Check sheet for the drawn part. Datum: minimum x, y, z corner. Units: mm. A direction names the side the tool comes from. Coordinates: 2 decimals unless noted, no trailing zeros. Loops run counter-clockwise (first coordinate to the right, second up) from the corner with the lowest first, then second, coordinate; pieces in that order, holes last. Notation, with made-up numbers: (-31.75, 49.5) - (-6.75, 49.5) arc R29 cw to (-6.75, 72.5) - close; hole circle Ø3 at (-29.5, 4). An arc over 180 degrees is marked (long way). Answer as CSV lines item,"result". Start each with the question number.
1. Set-up check for the marked faces 1, 2, 3, 4 and 5: record each of +Z, -Z, +X, -X, +Y, -Y from which the full face is reachable in a straight line by a thin tool's end or side.
2. Cross-section at D-D (z = 5). Enter the section's corners in (x, y).
3. Cross-section at C-C (x = 1.75). Enter the section's corners in (y, z), plus the area to 3 significant figures.
4. Release check for a two-part mould opening along Y. For the marked faces 6, 7 and 8 record: pulls with the +Y half, pulls with the -Y half, needs draft (parallel to the pull), parting line crosses it, or undercut.
5. Cross-section at B-B (y = 5). Enter the section's corners in (x, z).
6. Material ranges on line 1 (Y direction, x = 1.25, z = 12); line 2 (Z direction, x = 1.9, y = 11.25); line 3 (Y direction, x = 0.45, z = 5), recorded low to high. Write a range as [from, to].
7. Cross-section at A-A (z = 8.5). Enter the section's corners in (x, y).
8. Gauge pin test, flat ends, axial feed: P1, Ø1, axis at x = 1, z = 1, coming from the +Y side; P2, Ø0.6, axis at x = 1, y = 11, coming from the +Z side; P3, Ø4, axis at y = 10.5, z = 15, coming from the -X side; P4, Ø1, axis at x = 1, y = 15.5, coming from the -Z side. Record the tip position at first contact, or that the pin passes through.
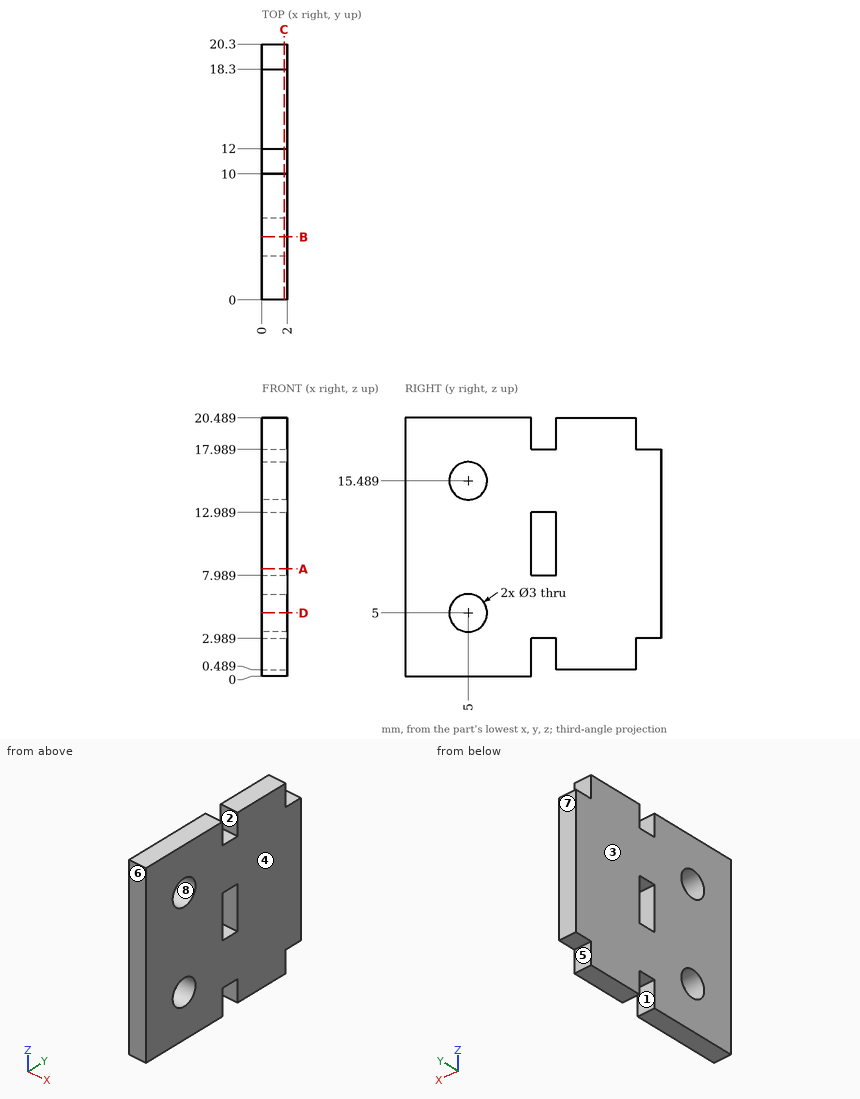
Values follow:
1,face 1,"-Z, +X, -X"
1,face 2,"+Z, +X, -X"
1,face 3,"+Z, -Z, -X, +Y, -Y"
1,face 4,"+Z, -Z, +X, +Y, -Y"
1,face 5,"-Z, +X, -X, +Y"
2,outline,"(0, 0) - (2, 0) - (2, 3.5) - (0, 3.5) - close; (0, 6.5) - (2, 6.5) - (2, 20.3) - (0, 20.3) - close"
3,outline,"(0, 0) - (10, 0) - (10, 2.99) - (12, 2.99) - (12, 0.49) - (18.3, 0.49) - (18.3, 2.99) - (20.3, 2.99) - (20.3, 17.99) - (18.3, 17.99) - (18.3, 20.49) - (12, 20.49) - (12, 17.99) - (10, 17.99) - (10, 20.49) - (0, 20.49) - close; hole circle Ø3 at (5, 5); hole circle Ø3 at (5, 15.49); hole (10, 7.99) - (12, 7.99) - (12, 12.99) - (10, 12.99) - close"
3,area,"367 mm²"
4,face 6,"pulls with the -Y half"
4,face 7,"pulls with the +Y half"
4,face 8,"undercut"
5,outline,"(0, 0) - (2, 0) - (2, 3.5) - (0, 3.5) - close; (0, 6.5) - (2, 6.5) - (2, 13.99) - (0, 13.99) - close; (0, 16.99) - (2, 16.99) - (2, 20.49) - (0, 20.49) - close"
6,line 1,"y = [0, 10], [12, 20.3]"
6,line 2,"z = [2.99, 7.99], [12.99, 17.99]"
6,line 3,"y = [0, 3.5], [6.5, 20.3]"
7,outline,"(0, 0) - (2, 0) - (2, 10) - (0, 10) - close; (0, 12) - (2, 12) - (2, 20.3) - (0, 20.3) - close"
8,P1,"stops at y = 18.3"
8,P2,"stops at z = 17.99"
8,P3,"stops at x = 0"
8,P4,"stops at z = 0.49"
